from build123d import *

# Parameters (mm, degrees)
F1_DEPTH = 63.5
F2_DEPTH = 25.4
F0_W     = 25.4
F0_H     = 19.05
F3_DEPTH = 25.4
F4_DEPTH = 7.9375
F6_R     = 6.35


with BuildPart() as f1:
    # F0 (on Front) → F1 (new body, symmetric)
    with BuildSketch(Plane.XZ):
        Polygon((-41.275, 9.525), (-41.275, -9.525), (41.275, -9.525), (41.275, 9.525), (22.225, 9.525), align=None)
    extrude(amount=F1_DEPTH, both=True)

    # F0 (on Front) → F2 (join, symmetric)
    with BuildSketch(Plane.XZ):
        with BuildLine():
            Line((22.225, 9.525), (41.275, 9.525))
            Line((41.275, 9.525), (41.275, 27.0002))
            ThreePointArc((41.275, 27.0002), (45.9246798487, 38.2255201513), (57.15, 42.8752))
            Line((57.15, 42.8752), (60.325, 42.8752))
            Line((60.325, 42.8752), (60.325, 61.9252))
            Line((60.325, 61.9252), (57.15, 61.9252))
            add(Edge.make_bspline(
                [(54.0079160608, 61.7835715088), (55.0442891577, 61.8415102214), (56.0915997071, 61.8888238055), (57.15, 61.9252)],
                knots=[109.4395067018, 109.4395067018, 109.4395067018, 109.4395067018, 111.5045361635, 111.5045361635, 111.5045361635, 111.5045361635], degree=3))
            ThreePointArc((54.0079160608, 61.7835715088), (31.3673226121, 50.5588326367), (22.225, 27.0002))
            Line((22.225, 27.0002), (22.225, 9.525))
        make_face()
    extrude(amount=F2_DEPTH, both=True)

    # F0 (on Front) → F3 (join, symmetric)
    with BuildSketch(Plane.XZ):
        with Locations((73.025, 52.4002)):
            Rectangle(F0_W, F0_H)
    extrude(amount=F3_DEPTH, both=True)

    # F0 (on Front) → F4 (join, symmetric)
    with BuildSketch(Plane.XZ):
        with BuildLine():
            add(Edge.make_bspline(
                [(-41.275, 9.525), (-25.1212076231, 25.8003253275), (-0.9163175084, 58.7130176756), (54.0079160608, 61.7835715088)],
                knots=[0, 0, 0, 0, 109.4395067018, 109.4395067018, 109.4395067018, 109.4395067018], degree=3))
            Line((-41.275, 9.525), (22.225, 9.525))
            Line((22.225, 9.525), (22.225, 27.0002))
            ThreePointArc((22.225, 27.0002), (31.3673226121, 50.5588326367), (54.0079160608, 61.7835715088))
        make_face()
    extrude(amount=F4_DEPTH, both=True)

    # F0 (on Front) → F5 (revolve)
    with BuildSketch(Plane.XZ):
        Polygon((85.725, 66.675), (85.725, 61.9252), (85.725, 42.8752), (85.725, 38.1), (111.125, 38.1), (111.125, 66.675), align=None)
    revolve(axis=Axis((85.725, 0, 52.3875), (0, 0, -1)))

    # F6
    f6_edges = [f1.edges().sort_by_distance(p)[0] for p in [
        (41.275, -63.5, 0),
        (-41.275, -63.5, 0),
        (41.275, 63.5, 0),
        (-41.275, 63.5, 0),
    ]]
    fillet(f6_edges, radius=F6_R)


solid = f1.part
Design review of the part built by this model. Coordinates are the model's own, in mm. A direction names the side the tool comes from. Round coordinates to 2 decimals unless told otherwise and drop trailing zeros. Write each loop counter-clockwise with the first axis right and the second up, starting at its lowest first coordinate (ties: lowest second). Pieces come first, ordered by that corner, then holes. Notation, with made-up numbers: M -16,6 L 35,6 A14 ccw 35,20 Z; hole C -5,86.5 d10. An arc over 180 degrees is marked long. One line per item, written item: value. Start each with the question number.
1. Take a section at A-A on z = -4. State the section outline as (x, y) points (3 decimals).
2. To check wall thickness, follow probe 1 along Z at (x, y) = (74, -3) (3 decimals); probe 2 along Z at (x, y) = (9, 20.5) (3 decimals); probe 3 along Y at (x, z) = (2.5, 31.5). State the ranges of each line that lie inside material, in increasing order. Write a range as from..to.
3. Clearance check with flat-ended pins moving along their axes: P1, Ø4, axis at y = -5, z = 30.5, coming from the -X side; P2, Ø12, axis at x = 93.5, z = 49, coming from the -Y side; P3, Ø1, axis at y = -19.5, z = 32, coming from the +X side; P4, Ø8, axis at x = 96, y = 27, coming from the +Z side (3 decimals). State where each tip first meets the part, or that it passes through.
4. For faces 4 (the face through (7, -7.938, 30)), 5 (the face through (45.8, -0.4, 38.1)), 6 (the face through (86, 0, 38.1)), list the 3-axis set-ups (+Z, -Z, +X, -X, +Y, -Y) from which the entire face can be reached by the end or side of a thin tool; tool diameter is ignored.
5. Take a section at B-B on y = 38. State the section outline as (x, z) points (3 decimals).
6. Draft analysis for pull direction X (two halves, no side actions). For faces 1 (the face through (0, 63.5, 0)), 2 (the face through (60, 2, 42.875)), 3 (the face through (-41.275, -1, 0)), state which applies: pulls with the +X half, pulls with the -X half, needs draft (parallel to the pull), parting line crosses it, or undercut.
Computed:
1. outline: M -41.275,-57.15 A6.35 ccw -34.925,-63.5 L 34.925,-63.5 A6.35 ccw 41.275,-57.15 L 41.275,57.15 A6.35 ccw 34.925,63.5 L -34.925,63.5 A6.35 ccw -41.275,57.15 Z
2. probe 1: z = 38.1..66.675
2. probe 2: z = -9.525..9.525
2. probe 3: y = -7.94..7.94
3. P1: stops at x = -22.8
3. P2: stops at y = -25.34
3. P3: stops at x = 42.26
3. P4: stops at z = 66.675
4. face 4: +Z, -X, -Y
4. face 5: -Z, +Y, -Y
4. face 6: -Z, +X, +Y, -Y
5. outline: M -41.275,-9.525 L 41.275,-9.525 L 41.275,9.525 L -41.275,9.525 Z
6. face 1: needs draft
6. face 2: undercut
6. face 3: pulls with the -X half
